Design review of the part built by this model. Coordinates are the model's own, in mm. Face numbers are marked on the shaded views. A direction names the side the tool comes from. Coordinates: 2 decimals unless noted, no trailing zeros. Loops run counter-clockwise (first coordinate to the right, second up) from the corner with the lowest first, then second, coordinate; pieces in that order, holes last. Notation, with made-up numbers: (-5.75, -12) -> (31.25, -12) arc R17 cw to (31.25, 17) -> close; hole circle Ø6 at (45.5, 26). An arc over 180 degrees is marked (long way). Answer in a Markdown table with one row per item.
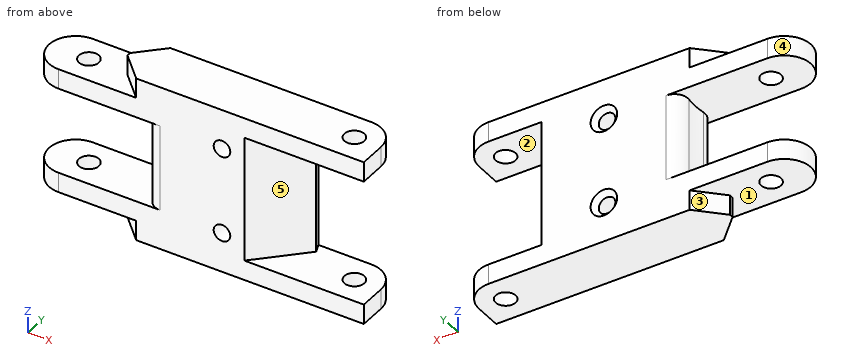
Autodesk Inventor part; units mm, degrees
ref_plane "YZ Plane" through (0, 0, 0) normal (1, 0, 0) x (0, 1, 0)
ref_plane "XZ Plane" through (0, 0, 0) normal (0, 1, 0) x (-1, 0, 0)
ref_plane "XY Plane" through (0, 0, 0) normal (0, 0, 1) x (1, 0, 0)
sketch "Skizze1" plane through (0, 0, 0) normal (0, 0, 1) x (1, 0, 0)
  circle A0 centre (0, 0) radius 4 construction
  circle A1 centre (40, 0) radius 4 construction
  line L0 (0, 0) -> (40, 0) construction
  arc A2 (0, 4) -> (0, -4) centre (0, 0) ccw
  arc A3 (44, 0) -> (40, 4) centre (40, 0) ccw
  line L1 (0, 4) -> (40, 4)
  line L2 (0, -4) -> (44, -4)
  line L3 (44, -4) -> (44, 0)
  dimension "d0" = 8
  dimension "d1" = 40
extrude "Extrusion1" add sketch "Skizze1" along normal blind 3
sketch "Skizze2" plane through (0, 0, 3) normal (0, 0, 1) x (1, 0, 0)
  arc A0 (0, 4) -> (0, -4) centre (0, 0) ccw
  line L0 (0, -4) -> (44, -4)
  line L1 (44, -4) -> (44, 0)
  arc A1 (44, 0) -> (40, 4) centre (40, 0) ccw
  line L2 (40, 4) -> (0, 4)
  line L3 (6, 4) -> (34, 4)
  line L4 (34, 4) -> (34, -4)
  line L5 (34, -4) -> (6, -4)
  line L6 (6, -4) -> (6, 4)
  line L7 (0, 0) -> (-4, 0) construction
  line L8 (-4, 0) -> (-4, -4) construction
  line L9 (-4, -4) -> (0, -4) construction
  line L10 (0, -4) -> (0, 0) construction
  dimension "d4" = 10
  dimension "d5" = 4
  dimension "d6" = 10
extrude "Extrusion2" add sketch "Skizze2" along normal blind 9.5 contours L2 L4 L0 L6
sketch "Skizze3" plane through (0, 0, 0) normal (0, 0, -1) x (-1, 0, 0)
  line L0 (-6, -4) -> (-6, 4)
  line L1 (-6, 4) -> (0, 4)
  arc A0 (0, -4) -> (0, 4) centre (0, 0) ccw
  line L2 (0, -4) -> (-6, -4)
sketch "Skizze4" plane through (0, 0, 3) normal (0, 0, 1) x (1, 0, 0)
  line L0 (6, -4) -> (6, 4)
  line L1 (6, 4) -> (0, 4)
  arc A0 (0, 4) -> (0, -4) centre (0, 0) ccw
  line L2 (0, -4) -> (6, -4)
extrude "Extrusion3" add sketch "Skizze4" along normal blind 3
extrude "Extrusion4" cut sketch "Skizze3" against normal blind 3
sketch "Skizze5" plane through (0, 0, 0) normal (0, 0, -1) x (-1, 0, 0)
  line L0 (-6, -4) -> (-6, 4)
  line L1 (-40, 4) -> (-6, 4)
  arc A0 (-40, 4) -> (-44, 0) centre (-40, 0) ccw
  line L2 (-6, -4) -> (-44, -4)
  line L3 (-6, 0.3) -> (-9.7, 4)
  line L4 (-9.7, -4) -> (-6, -0.3)
  line L5 (-9.7, 4) -> (-6, 4)
  line L6 (-6, 0.3) -> (-6, 4)
  line L7 (0, 0) -> (-40, 0) construction
  circle A1 centre (0, 0) radius 4
  line L8 (-6, -4) -> (-6, 4)
  line L9 (0, -4) -> (-6, -4)
  arc A2 (0, -4) -> (0, 4) centre (0, 0) ccw
  line L10 (-6, 4) -> (0, 4)
  line L11 (-3.0018, 2.6437) -> (3.0018, -2.6437)
  line L12 (3.0018, -2.6437) -> (-9.9619, -17.3635)
  line L13 (-9.9619, -17.3635) -> (-15.9655, -12.0761)
  line L14 (-15.9655, -12.0761) -> (-3.0018, 2.6437)
  dimension "d13" = 45
  dimension "d14" = 0.6
extrude "Extrusion5" cut sketch "Skizze5" against normal up to surface (3 mm away) contours L0 L14 L2 L4 | L3 L1 L0 | L0 L2 L14
mirror "Spiegeln1" about plane through (20, 0, 12.5) normal (0, 0, 1)
sketch "Skizze6" plane through (6, -4, 19) normal (0, 0, -1) x (-1, 0, 0)
  line L0 (0, 8) -> (0, 0)
  line L1 (6, 0) -> (0, 0)
  arc A0 (6, 0) -> (6, 8) centre (6, 4) ccw
  line L2 (0, 8) -> (6, 8)
  line L3 (-3.7, 0) -> (-38, 0)
  line L4 (6, 0) -> (-3.7, 0)
  line L5 (0, 3.7) -> (-3.7, 0)
  line L6 (0, 3.7) -> (0, 4.3)
  line L7 (-3.7, 8) -> (0, 4.3)
  line L8 (-3.7, 8) -> (6, 8)
  arc A1 (6, 0) -> (6, 8) centre (6, 4) ccw
extrude "Extrusion6" cut sketch "Skizze6" along normal up to surface (13 mm away) contours L0 L7 L8 | L0 L4 L5
sketch "Skizze7" plane through (0, 0, 19) normal (0, 0, -1) x (-1, 0, 0)
  arc A0 (0, -4) -> (0, 4) centre (0, 0) ccw
  circle A1 centre (0, 0) radius 11.4
  circle A2 centre (0, 0) radius 13 construction
  dimension "d19" = 1.6
  dimension "d47" = 26
extrude "Extrusion7" cut sketch "Skizze7" along normal up to surface (13 mm away)
sketch "Skizze8" plane through (44, -4, 22) normal (0, 0, -1) x (-1, 0, 0)
  line L0 (10, 8) -> (10, 0)
  line L1 (10, 0) -> (0, 0)
  line L2 (10, 8) -> (18, 0)
  line L3 (18, 0) -> (10, 0)
  point P0 (44, 4)
  dimension "d22" = 45
extrude "Extrusion8" cut sketch "Skizze8" along normal up to surface (19 mm away)
sketch "Skizze9" plane through (0, 0, 0) normal (0, 0, -1) x (-1, 0, 0)
  arc A0 (-40, 4) -> (-44, 0) centre (-40, 0) ccw
  point P0 (0, 0)
hole "Bohrung1" at (40, 0, 0) direction (0, 0, 1) diameter 3 end through all
hole "Bohrung2" at (0, 0, 0) direction (0, 0, 1) diameter 3 end through all
fillet "Rundung1" radius 2 2 edges at (10.6752, 4, 12.5) (10.6752, -4, 12.5)
chamfer "Fase1" distance 2 angle 45 1 edges at (34, 4, 12.5)
sketch "Skizze12" plane through (40, 4, 3) normal (0, 1, 0) x (1, 0, 0)
  line L0 (-8, 0) -> (-8, -19)
  line L1 (-26.7501, -3) -> (-8, -3)
  line L2 (-26.7501, -16) -> (-8, -16)
  point P0 (-40, 3)
  point P1 (-17.375, -3)
  point P2 (-17.375, -16)
  point P3 (-17.375, -3)
  point P4 (-17.375, -16)
hole "Bohrung3" at (22.625, 4, 6) at (22.625, 4, 19) direction (0, -1, 0) diameter 2.5 end through all countersink diameter 4 countersink angle 90
sketch "Skizze13" plane through (0, -4, 22) normal (0, 0, 1) x (1, 0, 0)
  line L0 (0, 0) -> (9.7, 0)
  line L1 (9.7, 8) -> (0, 8)
  arc A0 (0, 8) -> (0, 0) centre (0, 4) ccw
  arc A1 (-2, 8) -> (-2, 0) centre (-2, 4) ccw
  line L2 (-2, 8) -> (0, 8)
  line L3 (0, 0) -> (-2, 0)
  dimension "d59" = 2
extrude "Extrusion11" add sketch "Skizze13" against normal up to surface (3 mm away)
ref_plane "Arbeitsebene1" through (44, -4, 12.5) normal (0, 0, -1) x (-1, 0, 0)
mirror "Spiegeln2" about plane through (44, -4, 12.5) normal (0, 0, -1) of "Extrusion11"
equation "\"d0\" = Finger_diameter"
equation "\"d1\" = FingerLaenge_A"
equation "\"d2\" = FingerWall"
equation "\"d4\" = 2.5 * d5"
equation "\"d6\" = d4"
equation "\"d7\" = -0.5 * FingerWall + 0.5 * Finger_width"
equation "\"d9\" = FingerWall"
equation "\"d11\" = FingerWall"
equation "\"d15\" = FingerWall"
equation "\"d32\" = bearingHole"
equation "\"FingerLaenge_A\" = 40"
equation "\"FingerLaenge_B\" = 25"
equation "\"Hebel_B\" = 25"
equation "\"Finger_width\" = 22"
equation "\"Finger_diameter\" = 8"
equation "\"FingerWall\" = 3"
equation "\"Hebel_basis_2\" = 15"
equation "\"Join_width\" = 3"
equation "\"bearingHole\" = 3"
equation "\"bearingWall\" = 4"
equation "\"support_D\" = 0.25"
properties part number "FingerPartA"
(1) Take a section at C-C on x = 39. Give the boundary of the cut face in (y, z).
Evaluation:
| item | result |
|---|---|
| outline | (-4, 0) -> (-1.12, 0) -> (-1.12, 3) -> (-4, 3) -> close; (-4, 22) -> (-1.12, 22) -> (-1.12, 25) -> (-4, 25) -> close; (1.12, 0) -> (4, 0) -> (4, 3) -> (1.12, 3) -> close; (1.12, 22) -> (4, 22) -> (4, 25) -> (1.12, 25) -> close |
(2) Draft analysis for pull direction Z (two halves, no side actions). For the marked faces 1, 2 and 3, state which applies: pulls with the +Z half, pulls with the -Z half, needs draft (parallel to the pull), parting line crosses it, or undercut.
Evaluation:
| item | result |
|---|---|
| face 1 | pulls with the -Z half |
| face 2 | undercut |
| face 3 | needs draft |
(3) For pin 1 (3 mm diameter, centred on y = 1.5, z = 16, fed in from -X); pin 2 (2.5 mm diameter, centred on x = -0.5, y = -2, fed in from +Z); pin 3 (0.7 mm diameter, centred on y = 0, z = 23.5, fed in from -X), all flat-tipped, find the tip position at first contact; note any pin that passes through.
Evaluation:
| item | result |
|---|---|
| pin 1 | stops at x = 11.25 |
| pin 2 | stops at z = 22 |
| pin 3 | stops at x = 6 |
(4) Take a section at B-B on x = 0. Give the boundary of the cut face in (y, z), and give its area (3 significant figures).
Evaluation:
| item | result |
|---|---|
| outline | (-4, 3) -> (-1.5, 3) -> (-1.5, 6) -> (-4, 6) -> close; (-4, 19) -> (-1.5, 19) -> (-1.5, 22) -> (-4, 22) -> close; (1.5, 3) -> (4, 3) -> (4, 6) -> (1.5, 6) -> close; (1.5, 19) -> (4, 19) -> (4, 22) -> (1.5, 22) -> close |
| area | 30.0 mm² |
(5) To check wall thickness, follow probe 1 along Y at (x, z) = (0, 4.65); probe 2 along Z at (x, y) = (2, -0.5); probe 3 along Z at (x, y) = (10, 0). State the ranges of each line that lie inside material, in increasing order.
Evaluation:
| item | result |
|---|---|
| probe 1 | y = -4 to -1.5, 1.5 to 4 |
| probe 2 | z = 3 to 6, 19 to 22 |
| probe 3 | z = 0 to 6, 19 to 25 |
(6) Tool access review of the marked faces 4 and 5: name each direction out of +Z, -Z, +X, -X, +Y, -Y from which nothing blocks a thin tool from reaching the whole face with its end or side.
Evaluation:
| item | result |
|---|---|
| face 4 | +Z, -Z, -X |
| face 5 | +X, -Y |
(7) Take a section at A-A on x = 9. Give the boundary of the cut face in (y, z).
Evaluation:
| item | result |
|---|---|
| outline | (-4, 3) -> (-3.3, 3) -> (-3.3, 0) -> (3.3, 0) -> (3.3, 3) -> (4, 3) -> (4, 6) -> (-4, 6) -> close; (-4, 19) -> (4, 19) -> (4, 22) -> (3.3, 22) -> (3.3, 25) -> (-3.3, 25) -> (-3.3, 22) -> (-4, 22) -> close |
